The listing builds one solid part. Answer for the finished solid, in the listing's coordinates (mm). A direction names the side the tool comes from. Coordinates: 2 decimals unless noted, no trailing zeros. Write each loop counter-clockwise with the first axis right and the second up, starting at its lowest first coordinate (ties: lowest second). Pieces come first, ordered by that corner, then holes.
from build123d import *

# Parameters (mm, degrees)
IZIM1_W                     = 56
IZIM1_H                     = 75
Y_KSEKLIK_EKSTR_ZYON1_DEPTH = 18
IZIM3_R                     = 6
KES_EKSTR_ZYON1_DEPTH       = 96.315266353
IZIM4_W                     = 32
IZIM4_H                     = 5
KES_EKSTR_ZYON2_DEPTH       = 96.315266353
Y_KSEKLIK_EKSTR_ZYON2_DEPTH = 6
IZIM7_R                     = 11
Y_KSEKLIK_EKSTR_ZYON3_DEPTH = 23
FEDER1_REACH                = 134.194
IZIM8_WALL_W                = 310.68379038
IZIM8_WALL_H                = 12


with BuildPart() as part:
    # Çizim1 → Yükseklik-Ekstrüzyon1 (new body)
    with BuildSketch(Plane(origin=(0, 0, 0), x_dir=(1, 0, 0), z_dir=(0, 1, 0))):
        with Locations((28, -37.5)):
            Rectangle(IZIM1_W, IZIM1_H)
    extrude(amount=Y_KSEKLIK_EKSTR_ZYON1_DEPTH)

    # Çizim3 → Kes-Ekstrüzyon1 (cut, through all)
    with BuildSketch(Plane(origin=(0, 18, 0), x_dir=(1, 0, 0), z_dir=(0, 1, 0))):
        with Locations(Location((28, -15, 0), (0, 0, 270))):
            Circle(IZIM3_R)
        with Locations(Location((28, -60, 0), (0, 0, 270))):
            Circle(IZIM3_R)
    extrude(amount=-KES_EKSTR_ZYON1_DEPTH, mode=Mode.SUBTRACT)

    # Çizim4 → Kes-Ekstrüzyon2 (cut, through all)
    with BuildSketch(Plane.XY.offset(75)):
        with Locations((28, 2.5)):
            Rectangle(IZIM4_W, IZIM4_H)
    extrude(amount=-KES_EKSTR_ZYON2_DEPTH, mode=Mode.SUBTRACT)

    # Çizim5 → Yükseklik-Ekstrüzyon2 (add, symmetric)
    with BuildSketch(Plane.XY.offset(37.5)):
        Polygon((0, 18), (56, 18), (56, 63), align=None)
    extrude(amount=Y_KSEKLIK_EKSTR_ZYON2_DEPTH, both=True)

    # Çizim7 → Yükseklik-Ekstrüzyon3 (add)
    with BuildSketch(Plane(origin=(0, 63, 0), x_dir=(1, 0, 0), z_dir=(0, 1, 0))):
        with BuildLine():
            Line((56, -31.5), (75.029437252, -31.5))
            ThreePointArc((75.029437252, -31.5), (110, -37.5), (75.029437252, -43.5))
            Line((75.029437252, -43.5), (56, -43.5))
            Line((56, -43.5), (56, -37.5))
            Line((56, -37.5), (56, -31.5))
        make_face()
        with Locations(Location((92, -37.5, 0), (0, 0, 270))):
            Circle(IZIM7_R, mode=Mode.SUBTRACT)
    extrude(amount=-Y_KSEKLIK_EKSTR_ZYON3_DEPTH)

    # Çizim8 wall → Feder1 (add, up to next)
    with BuildSketch(Plane(origin=(65.514718626, 20, 37.5), x_dir=(0.42959895901, 0.903019786283, 0), z_dir=(-0.903019786283, 0.42959895901, 0)), mode=Mode.PRIVATE) as feder1_sk1:
        Rectangle(IZIM8_WALL_W, IZIM8_WALL_H)
    feder1_tool1 = extrude(feder1_sk1.sketch, amount=FEDER1_REACH, mode=Mode.PRIVATE) - part.part
    add(feder1_tool1.solids().sort_by_distance((65.514718626, 20, 37.5))[0])


solid = part.part
1. Section A-A on z = 15 is taken. Give the vertices of the cut face in (x, y), then the cut area to 3 significant figures.
Results found:
outline: (0, 0) - (12, 0) - (12, 5) - (22, 5) - (22, 18) - (0, 18) - close; (34, 5) - (44, 5) - (44, 0) - (56, 0) - (56, 18) - (34, 18) - close
area: 692 mm2
2. Section B-B on x = 92 is taken. Give the vertices of the cut face in (y, z), then the cut area to 3 significant figures.
Results found:
outline: (40, 19.5) - (63, 19.5) - (63, 26.5) - (40, 26.5) - close; (40, 48.5) - (63, 48.5) - (63, 55.5) - (40, 55.5) - close
area: 322 mm2
3. Section C-C on z = 29.5 is taken. Give the vertices of the cut face in (x, y).
Results found:
outline: (0, 0) - (12, 0) - (12, 5) - (44, 5) - (44, 0) - (56, 0) - (56, 18) - (0, 18) - close; (75.88, 40) - (84.45, 40) - (84.45, 63) - (75.88, 63) - close; (99.55, 40) - (108.12, 40) - (108.12, 63) - (99.55, 63) - close
4. Find the intervals of material crossed by L1, parallel to X at y = 10, z = 60; L2, parallel to Z at x = 33, y = 21.5; L3, parallel to Y at x = 35, z = 29.5, in increasing order.
Results found:
L1: x = 0 to 22, 34 to 56
L2: z = 31.5 to 43.5
L3: y = 5 to 18
5. Flat-ended cylindrical pins translate along their axes: P1, Ø4, axis at x = 90, z = 17, coming from the -Y side; P2, Ø8, axis at x = 42, y = 53.5, coming from the +Z side; P3, Ø14.5, axis at y = 6, z = 16.5, coming from the +X side; P4, Ø14, axis at x = 28, z = 60, coming from the -Y side. Find the tip coordinate at first contact, or state that the pin passes through.
Results found:
P1: passes through
P2: stops at z = 43.5
P3: stops at x = 56
P4: stops at y = 5
6. Section D-D on y = 14.5 is taken. Give the vertices of the cut face in (x, z).
Results found:
outline: (0, 0) - (56, 0) - (56, 31.5) - (62.9, 31.5) - (62.9, 43.5) - (56, 43.5) - (56, 75) - (0, 75) - close; hole circle Ø12 at (28, 15); hole circle Ø12 at (28, 60)
7. For a pull along Z with two mould halves and no side action, classify faces 1 (the cylindrical face through (22.677, 11.591, 17.769)), 2 (the flat face through (44, 2, 38)), 3 (the flat face through (28, 11, 0)) as pulls with the +Z half, pulls with the -Z half, needs draft (parallel to the pull), parting line crosses it, or undercut.
Results found:
face 1: undercut
face 2: needs draft
face 3: pulls with the -Z half
8. A tool of negligible diameter and unlimited length cuts with its end or side. For faces 4 (the flat face through (21, 18, 59)), 5 (the flat face through (12, 2, 38)), 6 (the flat face through (56, 9, 59)), 7 (the flat face through (101, 40, 45)), 8 (the flat face through (56, 9, 16)), from which of +Z, -Z, +X, -X, +Y, -Y can it reach the whole face along a straight path? Write none if from no direction.
Results found:
face 4: +Z, +X, -X, +Y
face 5: +Z, -Z, -Y
face 6: +Z, +X, +Y, -Y
face 7: +Z, -Z, +X, -Y
face 8: -Z, +X, +Y, -Y
